Can you work these out from the drawing? Everything is in mm from the part's minimum corner. A direction names the side the tool comes from. Round coordinates to 2 decimals unless told otherwise and drop trailing zeros. Write each loop counter-clockwise with the first axis right and the second up, starting at its lowest first coordinate (ties: lowest second). Pieces come first, ordered by that corner, then holes.
Q1. For the marked faces 1, 2 and 3, which set-ups out of +Z, -Z, +X, -X, +Y, -Y let a thin tool reach every point of the face, with its end or its side?
Q2. If we section it at A-A (z = 3): Please give me the cut outline in (x, y).
Q3. We'd pull the mould along Z, two halves only. Please class the marked faces 4, 5, 6 and 7: +Z half, -Z half, draft (parallel to the pull), parting line (faces both ways), or undercut.
Q4. I'm going to push a flat-ended pin straight in: pin 1 Ø1.5 at (x, z) = (36, 0.5) entering from +Y. Where does the tip first touch, or does it pass through?
Q5. If we section it at B-B (x = 50.5): Please give me the cut outline in (y, z), plus the area to 3 significant figures.
Q6. If we section it at C-C (z = 5.45): Please give me the cut outline in (x, y), plus the area to 3 significant figures.
Q7. If we section it at D-D (y = 5): Please give me the cut outline in (x, z).
Q8. Please list where these lines run through material, in increasing order: line 1 along Z through (x, y) = (50.5, 2.05); line 2 along Y through (x, z) = (7.5, 0.9); line 3 along X through (y, z) = (7, 2.35).
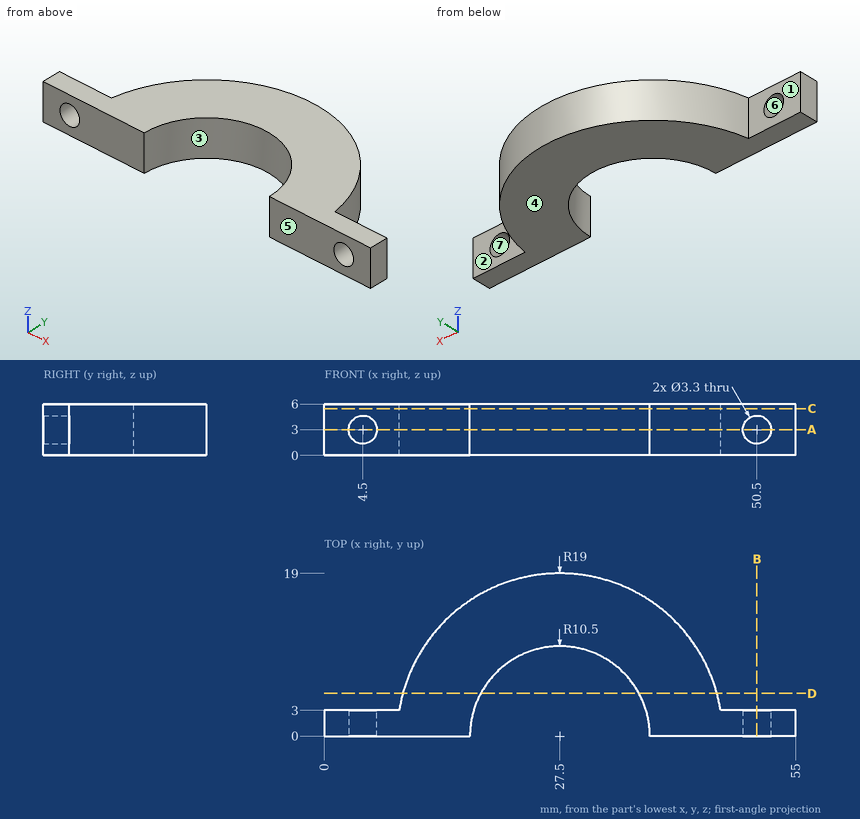
A:
1. face 1: +Z, -Z, -X, +Y
1. face 2: +Z, -Z, +X, +Y
1. face 3: +Z, -Z, -Y
2. outline: (0, 0) - (2.85, 0) - (2.85, 3) - (0, 3) - close; (6.15, 0) - (17, 0) arc R10.5 cw to (38, 0) - (48.85, 0) - (48.85, 3) - (46.26, 3) arc R19 ccw to (8.74, 3) - (6.15, 3) - close; (52.15, 0) - (55, 0) - (55, 3) - (52.15, 3) - close
3. face 4: -Z half
3. face 5: draft
3. face 6: undercut
3. face 7: undercut
4. pin 1: stops at y = 17.35
5. outline: (0, 0) - (3, 0) - (3, 1.35) - (0, 1.35) - close; (0, 4.65) - (3, 4.65) - (3, 6) - (0, 6) - close
5. area: 8.10 mm2
6. outline: (0, 0) - (17, 0) arc R10.5 cw to (38, 0) - (55, 0) - (55, 3) - (46.26, 3) arc R19 ccw to (8.74, 3) - (0, 3) - close
6. area: 445 mm2
7. outline: (9.17, 0) - (18.27, 0) - (18.27, 6) - (9.17, 6) - close; (36.73, 0) - (45.83, 0) - (45.83, 6) - (36.73, 6) - close
8. line 1: z = 0 to 1.35, 4.65 to 6
8. line 2: y = 0 to 3
8. line 3: x = 9.84 to 19.67, 35.33 to 45.16
